The listing builds one solid part. Answer for the finished solid, in the listing's coordinates (mm). Give positions to 0.01 mm unless a question says otherwise; leave off trailing zeros. Order: outer loops, then holes, each group sorted by start corner. A loop starts at its lowest first (then second) coordinate and runs counter-clockwise, first axis right, second up. Notation, with made-up numbers: (15.25, 3) - (57.25, 3) arc R13 cw to (57.25, 10) - close; hole circle Ø2 at (82, 31.25). An arc over 180 degrees is marked (long way). Answer as a JSON object with one key per item and string values. Group by question number.
Q1. A cutting plane is placed at A-A, the plane y = 638. Give the vertices of the cut face in (x, z), and give its area (3 significant figures).
Q2. Consider line 1 (X direction, y = 983.5, z = 0); line 2 (Z direction, x = 15, y = 990.75); line 3 (Z direction, x = 20.75, y = -815). Determine where each line is inside the solid, lowest interval first.
Q3. A cutting plane is placed at B-B, the plane z = 25.5. Give the vertices of the cut face in (x, y), and give its area (3 significant figures).
Q4. Given pin 1 (0.8 mm diameter, centred on x = 27, z = -94.5, fed in from +Y); pin 2 (15 mm diameter, centred on x = 14, z = 33.5, fed in from +Y); pin 3 (8 mm diameter, centred on x = 26, y = 100, fed in from -Z), each flat-ended and moving along its own axis, determine where each tip first touches the part or whether it passes through.
from build123d import *

# Parameters (mm, degrees)
F0_W      = 2000
F0_H      = 200
F1_DEPTH  = 30
F2_R      = 3
F3_DEPTH  = 30
F5_START  = -2
F4_W      = 10
F4_H      = 10
F5_DEPTH  = 1996
F6_R      = 3
F6_R_2    = 2.7931016095
F7_DEPTH  = 30
F8_W      = 10
F8_H      = 1
F9_DEPTH  = 2000
F10_D     = 5.1054
F10_DEPTH = 30
F10_TIP   = 1.5338169022
F11_D     = 5.1054
F11_DEPTH = 30
F11_TIP   = 1.5338169022


with BuildPart() as f1:
    # F0 (on Right) → F1 (new body)
    with BuildSketch(Plane.YZ):
        Rectangle(F0_W, F0_H)
    extrude(amount=F1_DEPTH)

    # F2 (on face) → F3 (join)
    with BuildSketch(Plane(origin=(0, 1000, 0), x_dir=(-1, 0, 0), z_dir=(0, 1, 0))):
        with Locations((-15, -50)):
            Circle(F2_R)
        with Locations((-15, 50)):
            Circle(F2_R)
    extrude(amount=F3_DEPTH)

    # F4 (on face) → F5 (join)
    with BuildSketch(Plane.XZ.offset(1000).offset(F5_START)):
        with Locations((15, -105)):
            Rectangle(F4_W, F4_H)
    extrude(amount=-F5_DEPTH)

    # F6 (on face) → F7 (join)
    with BuildSketch(Plane.XZ.offset(1000)):
        with Locations((15, 50)):
            Circle(F6_R)
        with Locations((15, -50)):
            Circle(F6_R_2)
    extrude(amount=F7_DEPTH)

    # F8 (on face) → F9 (cut)
    with BuildSketch(Plane.XZ.offset(998)):
        with Locations((25, -94.5)):
            Rectangle(F8_W, F8_H)
    extrude(amount=-F9_DEPTH, mode=Mode.SUBTRACT)

    # F10
    with Locations(Plane(origin=(0, 1000, 0), x_dir=(-1, 0, 0), z_dir=(0, 1, 0))):
        with Locations((-15, 0)):
            Hole(F10_D / 2, depth=F10_DEPTH)
            with Locations((0, 0, -(F10_DEPTH + F10_TIP / 2))):  # 118° drill point
                Cone(0, F10_D / 2, F10_TIP, mode=Mode.SUBTRACT)

    # F11
    with Locations(Plane.XZ.offset(1000)):
        with Locations((15, 0)):
            Hole(F11_D / 2, depth=F11_DEPTH)
            with Locations((0, 0, -(F11_DEPTH + F11_TIP / 2))):  # 118° drill point
                Cone(0, F11_D / 2, F11_TIP, mode=Mode.SUBTRACT)


solid = f1.part
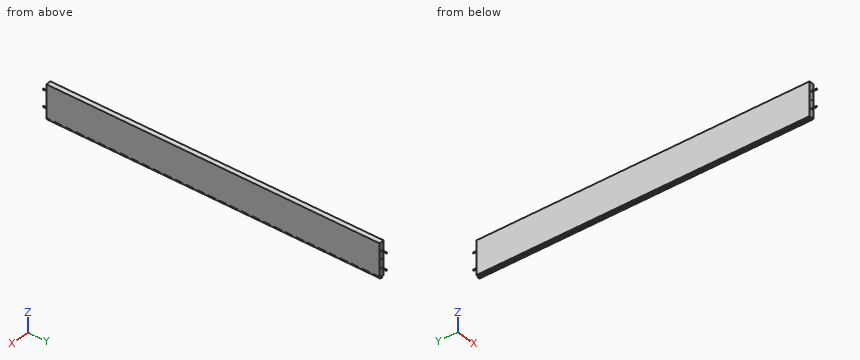
Reply:
{
 "1": {"outline": "(0, -100) - (10, -100) - (10, -110) - (20, -110) - (20, -100) - (30, -100) - (30, -95) - (20, -95) - (20, -94) - (30, -94) - (30, 100) - (0, 100) - close", "area": "6,090 mm^2"},
 "2": {"line 1": "x = 0 to 12.45, 17.55 to 30", "line 2": "z = -110 to -2.55, 2.55 to 100", "line 3": "z = -100 to -95, -94 to 100"},
 "3": {"outline": "(0, -1000) - (30, -1000) - (30, 1000) - (0, 1000) - close", "area": "60,000 mm^2"},
 "4": {"pin 1": "stops at y = -998", "pin 2": "stops at y = 1000", "pin 3": "stops at z = -100"}
}
